from build123d import *

# Parameters (mm, degrees)
F0_W     = 55.999888
F0_H     = 85.000084
F0_R     = 1.375
F1_DEPTH = 15.24
F2_R     = 3.499993


with BuildPart() as f1:
    # F0 (on Top) → F1 (new body)
    with BuildSketch(Plane.XY):
        with Locations((0, -10.000107)):
            Rectangle(F0_W, F0_H)
        with Locations((-24.499951, -28.999942)):
            Circle(F0_R, mode=Mode.SUBTRACT)
        with Locations((24.499951, -28.999942)):
            Circle(F0_R, mode=Mode.SUBTRACT)
        with Locations((-24.499951, 28.999942)):
            Circle(F0_R, mode=Mode.SUBTRACT)
        with Locations((24.499951, 28.999942)):
            Circle(F0_R, mode=Mode.SUBTRACT)
    extrude(amount=F1_DEPTH)

    # F2
    f2_edges = [f1.edges().sort_by_distance(p)[0] for p in [
        (-27.999944, 32.499935, 7.62),
        (27.999944, 32.499935, 7.62),
        (27.999944, -52.500149, 7.62),
        (-27.999944, -52.500149, 7.62),
    ]]
    fillet(f2_edges, radius=F2_R)


solid = f1.part
Could you check a few things on this model? Use its own coordinates, in mm. Round coordinates to 2 decimals unless told otherwise and drop trailing zeros. Put each result on its own line as item: value. Start each with the question number.
(1) Will this pin go through, and if not, where does the flat tip stop? pin 1 (2 mm diameter, centred on x = 24.5, y = -29, fed in from -Z).
(2) Thinking about a two-plate mould opening in Y: for faces 1 (the cylindrical face through (23.41, -29.84, 7.51)), 2 (the cylindrical face through (-25.51, 29.93, 7.51)), 3 (the cylindrical face through (26.95, 31.5, 7.73)), 4 (the flat face through (-28, -11, 8)), which applies, released by +Y, released by -Y, zero draft, split by the parting line, or undercut?
(3) I need wall thicknesses on probe 1 along Y at (x, z) = (-23.5, 11.75); probe 2 along Y at (x, z) = (-24, 2). Which ranges of each line are inside material? Lowest first, please.
Here are the results:
1. pin 1: passes through
2. face 1: undercut
2. face 2: undercut
2. face 3: released by +Y
2. face 4: zero draft
3. probe 1: y = -52.5 to -29.94, -28.06 to 28.06, 29.94 to 32.5
3. probe 2: y = -52.5 to -30.28, -27.72 to 27.72, 30.28 to 32.5
